from build123d import *

# Parameters (mm, degrees)
SKETCH1_W           = 80
SKETCH1_H           = 20
SKETCH1_R           = 2.25
BOSS_EXTRUDE1_DEPTH = 5
SKETCH2_W           = 80
SKETCH2_H           = 70
BOSS_EXTRUDE2_DEPTH = 5
SKETCH3_W           = 80
SKETCH3_H           = 20
SKETCH3_R           = 2.75
BOSS_EXTRUDE3_DEPTH = 5


with BuildPart() as part:
    # Sketch1 → Boss-Extrude1 (new body)
    with BuildSketch(Plane.XY):
        with Locations((40, 10)):
            Rectangle(SKETCH1_W, SKETCH1_H)
        with Locations((9, 10)):
            Circle(SKETCH1_R, mode=Mode.SUBTRACT)
        with Locations(Location((71, 10, 0), (0, 0, 180))):
            Circle(SKETCH1_R, mode=Mode.SUBTRACT)
    extrude(amount=BOSS_EXTRUDE1_DEPTH)

    # Sketch2 → Boss-Extrude2 (add)
    with BuildSketch(Plane.XZ):
        with Locations((40, 35)):
            Rectangle(SKETCH2_W, SKETCH2_H)
    extrude(amount=BOSS_EXTRUDE2_DEPTH)

    # Sketch3 → Boss-Extrude3 (add)
    with BuildSketch(Plane.XY.offset(70)):
        with Locations((40, 10)):
            Rectangle(SKETCH3_W, SKETCH3_H)
        with Locations((9, 10)):
            Circle(SKETCH3_R, mode=Mode.SUBTRACT)
        with Locations(Location((71, 10, 0), (0, 0, 180))):
            Circle(SKETCH3_R, mode=Mode.SUBTRACT)
    extrude(amount=-BOSS_EXTRUDE3_DEPTH)


solid = part.part
Geometry: final body of the model. Coordinates: model frame, mm. A direction names the side the tool comes from. Give positions to 0.01 mm unless a question says otherwise; leave off trailing zeros. Loops run counter-clockwise (first coordinate to the right, second up) from the corner with the lowest first, then second, coordinate; pieces in that order, holes last. Notation, with made-up numbers: (-33.5, 42) - (19.5, 42) arc R26 ccw to (19.5, 62) - close; hole circle Ø5 at (79, 37). An arc over 180 degrees is marked (long way). Answer as CSV lines item,"result". Start each with the question number.
1. Pin query (flat end, axial travel): P1, Ø7, axis at x = 71, y = 10, coming from the +Z side; P2, Ø8, axis at x = 46.5, z = 17, coming from the +Y side; P3, Ø5, axis at x = 71, y = 10, coming from the +Z side. Return the tip coordinate at first contact, or that it passes through.
2. Section D-D, the plane z = 11.5. Return loops of the section in (x, y).
3. Reachability of faces 5 (the face through (39, -5, 35)), 6 (the face through (39, 0, 35)), 7 (the face through (8.642, 12.727, 67.535)) from +Z, -Z, +X, -X, +Y, -Y: full face, straight path, thin tool, end or side. Return the list, or none.
4. Section A-A, the plane x = 9. Return loops of the section in (y, z), plus the area to 3 significant figures.
5. Section B-B, the plane y = 10. Return loops of the section in (x, z).
6. Draft query along Z for faces 1 (the face through (39, 8, 0)), 2 (the face through (80, -1, 35)), 3 (the face through (39, 10, 5)), 4 (the face through (39, 10, 65)). Return one class per face: released by +Z, released by -Z, zero draft, split by the parting line, or undercut.
7. Section C-C, the plane y = 15.75. Return loops of the section in (x, z).
8. Ray query, L1, parallel to Z at x = 66.5, y = 8.25; L2, parallel to Y at x = 9, z = 1.1; L3, parallel to Y at x = 71, z = 66.75. Return the intervals inside material, ascending.
Answers:
1,P1,"stops at z = 70"
1,P2,"stops at y = 0"
1,P3,"stops at z = 5"
2,outline,"(0, -5) - (80, -5) - (80, 0) - (0, 0) - close"
3,face 5,"+Z, -Z, +X, -X, -Y"
3,face 6,"+X, -X, +Y"
3,face 7,"+Z"
4,outline,"(-5, 0) - (7.75, 0) - (7.75, 5) - (0, 5) - (0, 65) - (7.25, 65) - (7.25, 70) - (-5, 70) - close; (12.25, 0) - (20, 0) - (20, 5) - (12.25, 5) - close; (12.75, 65) - (20, 65) - (20, 70) - (12.75, 70) - close"
4,area,"500 mm2"
5,outline,"(0, 0) - (6.75, 0) - (6.75, 5) - (0, 5) - close; (0, 65) - (6.25, 65) - (6.25, 70) - (0, 70) - close; (11.25, 0) - (68.75, 0) - (68.75, 5) - (11.25, 5) - close; (11.75, 65) - (68.25, 65) - (68.25, 70) - (11.75, 70) - close; (73.25, 0) - (80, 0) - (80, 5) - (73.25, 5) - close; (73.75, 65) - (80, 65) - (80, 70) - (73.75, 70) - close"
6,face 1,"released by -Z"
6,face 2,"zero draft"
6,face 3,"undercut"
6,face 4,"undercut"
7,outline,"(0, 0) - (80, 0) - (80, 5) - (0, 5) - close; (0, 65) - (80, 65) - (80, 70) - (0, 70) - close"
8,L1,"z = 0 to 5, 65 to 70"
8,L2,"y = -5 to 7.75, 12.25 to 20"
8,L3,"y = -5 to 7.25, 12.75 to 20"
